CAD build for the part. Positions are in the model's coordinates, mm. A direction names the side the tool comes from. Coordinates: 2 decimals unless noted, no trailing zeros. Loops run counter-clockwise (first coordinate to the right, second up) from the corner with the lowest first, then second, coordinate; pieces in that order, holes last. Notation, with made-up numbers: (88, 80) - (118, 80) arc R34 cw to (118, 112) - close; hole circle Ø8 at (7.25, -8). An arc over 180 degrees is marked (long way). Put each result on its own line as item: value.
```python
from build123d import *

# Parameters (mm, degrees)
SKETCH_1_R      = 1.5
SKETCH_1_R_2    = 5
EXTRUDE_1_DEPTH = 1.5


with BuildPart() as part:
    # 草圖1 → 填料-伸長1 (new body)
    with BuildSketch(Plane(origin=(0, 0, 0), x_dir=(1, 0, 0), z_dir=(0, 1, 0))):
        with BuildLine():
            Line((0, -3.980931511), (12.319060855, 2.328849967))
            ThreePointArc((12.319060855, 2.328849967), (14.431141465, 4.388450613), (15.014493405, 7.28025625))
            ThreePointArc((15.014493405, 7.28025625), (11.971039141, 65.394509034), (14.52184689, 123.53246884))
            ThreePointArc((14.52184689, 123.53246884), (15.377876917, 128.098069479), (17.067022361, 132.425226083))
            ThreePointArc((17.067022361, 132.425226083), (16.965589985, 149.77375384), (2.866920195, 159.883611111))
            ThreePointArc((2.866920195, 159.883611111), (0, 162), (-2.866920195, 159.883611111))
            ThreePointArc((-2.866920195, 159.883611111), (-16.965589985, 149.77375384), (-17.067022361, 132.425226083))
            ThreePointArc((-17.067022361, 132.425226083), (-15.377876917, 128.098069479), (-14.52184689, 123.53246884))
            ThreePointArc((-14.52184689, 123.53246884), (-11.971039141, 65.394509034), (-15.014493405, 7.28025625))
            ThreePointArc((-15.014493405, 7.28025625), (-14.431141465, 4.388450613), (-12.319060855, 2.328849967))
            Line((-12.319060855, 2.328849967), (0, -3.980931511))
        make_face()
        with Locations(Location((-12, 127.583592135, 0), (0, 0, 270))):
            Circle(SKETCH_1_R, mode=Mode.SUBTRACT)
        with Locations(Location((12, 127.583592135, 0), (0, 0, 270))):
            Circle(SKETCH_1_R, mode=Mode.SUBTRACT)
        with Locations(Location((8.6, 68.325395665, 0), (0, 0, 270))):
            Circle(SKETCH_1_R, mode=Mode.SUBTRACT)
        with Locations(Location((-8.6, 68.325395665, 0), (0, 0, 270))):
            Circle(SKETCH_1_R, mode=Mode.SUBTRACT)
        with Locations(Location((10.05, 6, 0), (0, 0, 270))):
            Circle(SKETCH_1_R, mode=Mode.SUBTRACT)
        with Locations(Location((-10.05, 6, 0), (0, 0, 270))):
            Circle(SKETCH_1_R, mode=Mode.SUBTRACT)
        with Locations(Location((0, 159, 0), (0, 0, 270))):
            Circle(SKETCH_1_R, mode=Mode.SUBTRACT)
        with Locations(Location((0, 0, 0), (0, 0, 270))):
            Circle(SKETCH_1_R, mode=Mode.SUBTRACT)
        with Locations(Location((0, 141, 0), (0, 0, 270))):
            Circle(SKETCH_1_R_2, mode=Mode.SUBTRACT)
        Polygon((0, 14.042409585), (-4.491071946, 11.449487988), (-5.101164168, 5.002829556), (5.101164168, 5.002829556), (4.491071946, 11.449487988), align=None, mode=Mode.SUBTRACT)
        with BuildLine():
            Line((0, 112.532142135), (-6.334048162, 108.875177723))
            ThreePointArc((-6.334048162, 108.875177723), (-6.614696141, 112.870067669), (-6.92146425, 116.863036776))
            Line((-6.92146425, 116.863036776), (-0.136378432, 120.780407899))
            ThreePointArc((-0.136378432, 120.780407899), (0, 120.816950389), (0.136378432, 120.780407899))
            Line((0.136378432, 120.780407899), (6.92146425, 116.863036776))
            ThreePointArc((6.92146425, 116.863036776), (6.614696141, 112.870067669), (6.334048162, 108.875177723))
            Line((6.334048162, 108.875177723), (0, 112.532142135))
        make_face(mode=Mode.SUBTRACT)
        with BuildLine():
            Line((0, 102.344922167), (5.753985291, 99.02285721))
            ThreePointArc((5.753985291, 99.02285721), (5.547257407, 94.643430297), (5.371890331, 90.262635518))
            Line((5.371890331, 90.262635518), (0, 93.364097846))
            Line((0, 93.364097846), (-5.371890331, 90.262635518))
            ThreePointArc((-5.371890331, 90.262635518), (-5.547257407, 94.643430297), (-5.753985291, 99.02285721))
            Line((-5.753985291, 99.02285721), (0, 102.344922167))
        make_face(mode=Mode.SUBTRACT)
        with BuildLine():
            Line((0, 84.072725452), (5.10712289, 81.124126676))
            ThreePointArc((5.10712289, 81.124126676), (5.026699976, 76.609736924), (4.97956534, 72.094876904))
            Line((4.97956534, 72.094876904), (0, 74.969830293))
            Line((0, 74.969830293), (-4.97956534, 72.094876904))
            ThreePointArc((-4.97956534, 72.094876904), (-5.026699976, 76.609736924), (-5.10712289, 81.124126676))
            Line((-5.10712289, 81.124126676), (0, 84.072725452))
        make_face(mode=Mode.SUBTRACT)
        with BuildLine():
            Line((0, 65.619773758), (4.987851065, 62.740036603))
            ThreePointArc((4.987851065, 62.740036603), (5.046332025, 58.016878131), (5.141244155, 53.29431128))
            Line((5.141244155, 53.29431128), (0, 56.262609977))
            Line((0, 56.262609977), (-5.141244155, 53.29431128))
            ThreePointArc((-5.141244155, 53.29431128), (-5.046332025, 58.016878131), (-4.987851065, 62.740036603))
            Line((-4.987851065, 62.740036603), (0, 65.619773758))
        make_face(mode=Mode.SUBTRACT)
        with BuildLine():
            Line((0, 46.827706802), (5.447027498, 43.68286401))
            ThreePointArc((5.447027498, 43.68286401), (5.648052955, 39.057684109), (5.884040018, 34.434156186))
            Line((5.884040018, 34.434156186), (0, 37.831308275))
            Line((0, 37.831308275), (-5.884040018, 34.434156186))
            ThreePointArc((-5.884040018, 34.434156186), (-5.648052955, 39.057684109), (-5.447027498, 43.68286401))
            Line((-5.447027498, 43.68286401), (0, 46.827706802))
        make_face(mode=Mode.SUBTRACT)
        with BuildLine():
            Line((0, 28.460830008), (6.494782795, 24.711065414))
            ThreePointArc((6.494782795, 24.711065414), (6.852315766, 19.927479382), (7.247310233, 15.146840877))
            Line((7.247310233, 15.146840877), (0, 19.331077391))
            Line((0, 19.331077391), (-7.247310233, 15.146840877))
            ThreePointArc((-7.247310233, 15.146840877), (-6.852315766, 19.927479382), (-6.494782795, 24.711065414))
            Line((-6.494782795, 24.711065414), (0, 28.460830008))
        make_face(mode=Mode.SUBTRACT)
        with BuildLine():
            Line((-6.717514421, 145.596194078), (-9.545941546, 148.424621202))
            ThreePointArc((-9.545941546, 148.424621202), (-9.545941546, 150.545941546), (-7.424621202, 150.545941546))
            Line((-7.424621202, 150.545941546), (-4.596194078, 147.717514421))
            ThreePointArc((-4.596194078, 147.717514421), (-4.596194078, 145.596194078), (-6.717514421, 145.596194078))
        make_face(mode=Mode.SUBTRACT)
        with BuildLine():
            Line((6.717514421, 145.596194078), (9.545941546, 148.424621202))
            ThreePointArc((9.545941546, 148.424621202), (9.545941546, 150.545941546), (7.424621202, 150.545941546))
            Line((7.424621202, 150.545941546), (4.596194078, 147.717514421))
            ThreePointArc((4.596194078, 147.717514421), (4.596194078, 145.596194078), (6.717514421, 145.596194078))
        make_face(mode=Mode.SUBTRACT)
        with BuildLine():
            Line((-4.596194078, 134.282485579), (-7.424621202, 131.454058454))
            ThreePointArc((-7.424621202, 131.454058454), (-9.545941546, 131.454058454), (-9.545941546, 133.575378798))
            Line((-9.545941546, 133.575378798), (-6.717514421, 136.403805922))
            ThreePointArc((-6.717514421, 136.403805922), (-4.596194078, 136.403805922), (-4.596194078, 134.282485579))
        make_face(mode=Mode.SUBTRACT)
        with BuildLine():
            Line((4.596194078, 134.282485579), (7.424621202, 131.454058454))
            ThreePointArc((7.424621202, 131.454058454), (9.545941546, 131.454058454), (9.545941546, 133.575378798))
            Line((9.545941546, 133.575378798), (6.717514421, 136.403805922))
            ThreePointArc((6.717514421, 136.403805922), (4.596194078, 136.403805922), (4.596194078, 134.282485579))
        make_face(mode=Mode.SUBTRACT)
    extrude(amount=EXTRUDE_1_DEPTH)


solid = part.part
```
Q1. Slice it at B-B, the plane y = 0.7. State how many separate pieces and enclosed holes the cut face has, then the cut area to 3 significant figures.
Determined:
separate pieces: 1
enclosed holes: 20
area: 3,480 mm2
Q2. Slice it at A-A, the plane z = 0. Give the cut face in (x, y), then the cut area to 3 significant figures.
Determined:
outline: (-7.77, 0) - (-1.5, 0) - (-1.5, 1.5) - (-7.77, 1.5) - close; (1.5, 0) - (7.77, 0) - (7.77, 1.5) - (1.5, 1.5) - close
area: 18.8 mm2
Q3. Tool access for faces 1 (the flat face through (-2.92, 0.74, -100.66)), 2 (the cylindrical face through (-11.97, 0.74, -66.21)): list every direction of +Z, -Z, +X, -X, +Y, -Y with a clear straight run to the whole face (end or side of a thin tool).
Determined:
face 1: +Y, -Y
face 2: -X, +Y, -Y
Q4. Wall check: L1, parallel to Z at x = -8, y = 0.3; L2, parallel to X at y = 0.6, z = -134; L3, parallel to X at y = 0.15, z = -77. Give the ranges that are in metal, low to high. Write a range as from..to.
Determined:
L1: -158.34..-150.9, -146.88..-135.12, -131.1..-69.7, -66.95..-0.12
L2: -17.77..-9.12, -4.88..4.88, 9.12..17.77
L3: -12.03..-5.03, 5.03..12.03
Q5. Pin check, flat tips, straight feed: pin 1 Ø6 at (x, z) = (6, -133) entering from +Y; pin 2 Ø2.5 at (x, z) = (0, 0) entering from -Y. Stop position of each tip, or through.
Determined:
pin 1: y = 1.5
pin 2: through
Q6. Slice it at C-C, the plane z = -42. Give the cut face in (x, y).
Determined:
outline: (-12.52, 0) - (-5.52, 0) - (-5.52, 1.5) - (-12.52, 1.5) - close; (5.52, 0) - (12.52, 0) - (12.52, 1.5) - (5.52, 1.5) - close
Q7. Mould opens along Z. For faces 3 (the flat face through (6.07, 0.74, 0.87)), 4 (the cylindrical face through (9.14, 0.74, -7.19)), 5 (the cylindrical face through (-8.149, 0.74, -66.895)) say: +Z half, -Z half, draft (parallel to the pull), parting line (faces both ways), or undercut.
Determined:
face 3: +Z half
face 4: undercut
face 5: undercut
